Read the model definition and answer for the solid it produces. Units are mm, in the model's axes. Face numbers are marked on the shaded views. A direction names the side the tool comes from. Coordinates: 2 decimals unless noted, no trailing zeros. Write each loop counter-clockwise with the first axis right and the second up, starting at its lowest first coordinate (ties: lowest second). Pieces come first, ordered by that corner, then holes. Notation, with made-up numbers: (-6, -28) -> (48, -28) arc R25 ccw to (48, 11) -> close; hole circle Ø1 at (4, -8.5). An arc over 180 degrees is marked (long way). Write item = value, one per line. Start each with the question number.
1) Section A-A (z = 0) is taken. Determine the outline of the cut face in (x, y), plus the area to 3 significant figures.
2) Section D-D (y = 3.5) is taken. Determine the outline of the cut face in (x, z).
3) Find the intervals of material crossed by line 1 along Y through (x, z) = (-1, 1.5); line 2 along X through (y, z) = (17, -2.5); line 3 along X through (y, z) = (8.5, -0.75), in increasing order. Write a range as from..to.
4) Flat-ended cylindrical pins translate along their axes: pin 1 Ø4 at (x, z) = (-2, -0.5) entering from +Y; pin 2 Ø2 at (y, z) = (11, -1.5) entering from +X; pin 3 Ø1 at (y, z) = (26.5, 1.5) entering from +X. Find the tip coordinate at first contact, or state that the pin passes through.
5) Section B-B (x = 0) is taken. Determine the outline of the cut face in (y, z), plus the area to 3 significant figures.
6) Section C-C (y = 23.5) is taken. Determine the outline of the cut face in (x, z), plus the area to 3 significant figures.
7) A tool of negligible diameter and unlimited length cuts with its end or side. For the marked faces 1, 2 and 3, from which of +Z, -Z, +X, -X, +Y, -Y can it reach the whole face along a straight path? Write none if from no direction.
from build123d import *

# Parameters (mm, degrees)
SKETCH1_W = 3.4544
SKETCH1_H = 30.988
SKETCH2_W = 1.7272
SKETCH2_H = 4.318
SKETCH3_W = 1.7272
SKETCH3_H = 4.318


with BuildPart() as part:
    # Sketch1 → Revolve1 (revolve)
    with BuildSketch(Plane.XY):
        with Locations((1.7272, 15.494)):
            Rectangle(SKETCH1_W, SKETCH1_H)
    revolve(axis=Axis((0, 0, 0), (0, 1, 0)))

    # Sketch2 → Cut-Revolve1 (revolve, cut)
    with BuildSketch(Plane.XY):
        with Locations((2.5908, 2.159)):
            Rectangle(SKETCH2_W, SKETCH2_H)
    revolve(axis=Axis((0, 0, 0), (0, 1, 0)), mode=Mode.SUBTRACT)

    # Sketch3 → Cut-Revolve2 (revolve, cut)
    with BuildSketch(Plane.XY):
        with Locations((2.5908, 28.829)):
            Rectangle(SKETCH3_W, SKETCH3_H)
    revolve(axis=Axis((0, 26.67, 0), (0, 1, 0)), mode=Mode.SUBTRACT)


solid = part.part
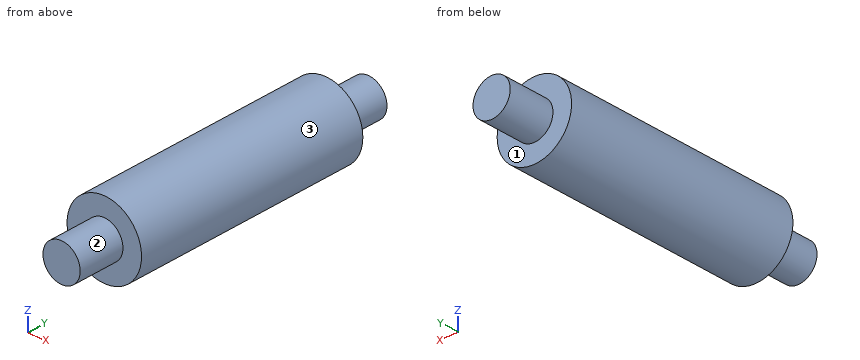
Answer key:
q1.outline = (-3.45, 4.32) -> (-1.73, 4.32) -> (-1.73, 0) -> (1.73, 0) -> (1.73, 4.32) -> (3.45, 4.32) -> (3.45, 26.67) -> (1.73, 26.67) -> (1.73, 30.99) -> (-1.73, 30.99) -> (-1.73, 26.67) -> (-3.45, 26.67) -> close
q1.area = 184 mm^2
q2.outline = circle Ø3.45 at (0, 0)
q3.line_1 = 4.32..26.67
q3.line_2 = -2.38..2.38
q3.line_3 = -3.37..3.37
q4.pin_1 = 30.99
q4.pin_2 = 3.42
q4.pin_3 = 3.31
q5.outline = (0, -1.73) -> (4.32, -1.73) -> (4.32, -3.45) -> (26.67, -3.45) -> (26.67, -1.73) -> (30.99, -1.73) -> (30.99, 1.73) -> (26.67, 1.73) -> (26.67, 3.45) -> (4.32, 3.45) -> (4.32, 1.73) -> (0, 1.73) -> close
q5.area = 184 mm^2
q6.outline = circle Ø6.91 at (0, 0)
q6.area = 37.5 mm^2
q7.face_1 = +Y
q7.face_2 = -Y
q7.face_3 = +Y, -Y
